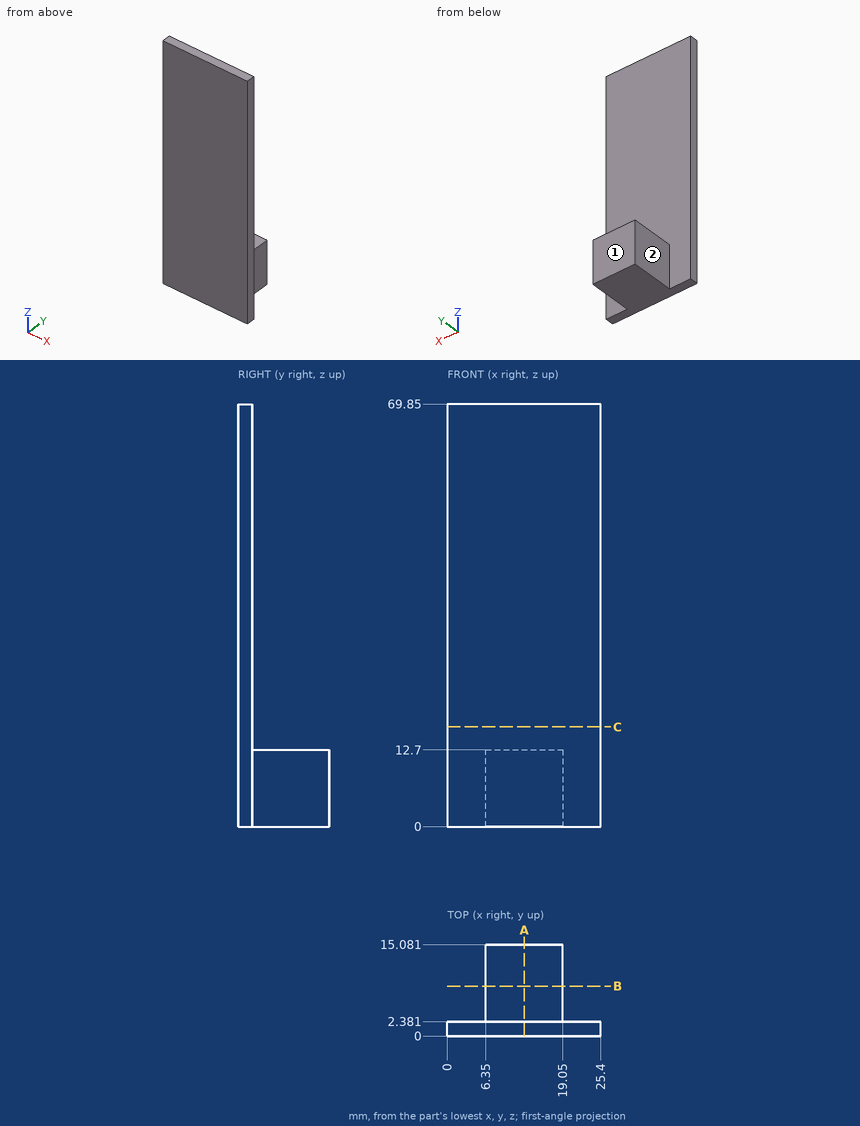
Part print with two shaded views. Sizes in mm from the minimum x, y, z corner. A direction names the side the tool comes from. Coordinates: 2 decimals unless noted, no trailing zeros. Write each loop counter-clockwise with the first axis right and the second up, starting at its lowest first coordinate (ties: lowest second). Pieces come first, ordered by that corner, then holes.
1. Band-saw the part on A-A, the plane x = 12.75. Give the cut face in (y, z), and give its area (3 significant figures).
Answer block:
outline: (0, 0) - (15.08, 0) - (15.08, 12.7) - (2.38, 12.7) - (2.38, 69.85) - (0, 69.85) - close
area: 328 mm2
2. Drill centre lines: probe 1 along Y at (x, z) = (11.5, 60.5); probe 2 along Z at (x, y) = (13.5, 8.5); probe 3 along X at (y, z) = (10.5, 7). Where is each one in solid material? Low to high.
Answer block:
probe 1: y = 0 to 2.38
probe 2: z = 0 to 12.7
probe 3: x = 6.35 to 19.05
3. 3-axis set-ups, long thin cutter, end or side, ignore diameter. For the marked faces 1 and 2: which of +Z, -Z, +X, -X, +Y, -Y reach the whole face in a straight line?
Answer block:
face 1: +Z, -Z, +X, -X, +Y
face 2: +Z, -Z, -X, +Y
4. Band-saw the part on B-B, the plane y = 8.25. Give the cut face in (x, z).
Answer block:
outline: (6.35, 0) - (19.05, 0) - (19.05, 12.7) - (6.35, 12.7) - close
5. Band-saw the part on C-C, the plane z = 16.5. Give the cut face in (x, y), and give its area (3 significant figures).
Answer block:
outline: (0, 0) - (25.4, 0) - (25.4, 2.38) - (0, 2.38) - close
area: 60.5 mm2
6. Drop flat-ended pins along their axis: pin 1 (8 mm diameter, centred on y = 5.5, z = 57, fed in from -X); pin 2 (7.5 mm diameter, centred on x = 14.5, z = 30.5, fed in from +Y); pin 3 (2 mm diameter, centred on x = 12, y = 9.5, fed in from +Z). Give the stop position or say it passes through.
Answer block:
pin 1: stops at x = 0
pin 2: stops at y = 2.38
pin 3: stops at z = 12.7
